Build history of the part. All positions in model axes, mm. A direction names the side the tool comes from. Coordinates: 2 decimals unless noted, no trailing zeros. Order: outer loops, then holes, each group sorted by start corner. A loop starts at its lowest first (then second) coordinate and runs counter-clockwise, first axis right, second up. Notation, with made-up numbers: (80.25, 84) -> (94.25, 84) arc R21 cw to (94.25, 91) -> close; hole circle Ø9 at (82.25, 81). An arc over 180 degrees is marked (long way). Write each question's results on one line, items separated by ' | '.
from build123d import *

# Parameters (mm, degrees)
F0_W         = 6
F0_H         = 10
F1_DEPTH     = 8
F2_T         = 1.2
F3_T1_DEPTH  = 6
F3_T3_DEPTH  = 10
F3_T9_DEPTH  = 8.2404819853
F3_T13_DEPTH = 12.2404819853
F3_T20_DEPTH = 8.2404819853
F3_T24_DEPTH = 12.2404819853
F3_T31_DEPTH = 12.2404819853
F3_T35_DEPTH = 8.2404819853
F3_T42_DEPTH = 8.2404819853
F3_T46_DEPTH = 12.2404819853


# Not quite as in the source:
# - a fillet or chamfer that OpenCascade refuses, or shapes differently, is made with other operations: its cross-section is extruded or revolved along the edge and cut away or added


with BuildPart() as f1:
    # F0 (on Top) → F1 (new body)
    with BuildSketch(Plane.XY):
        Rectangle(F0_W, F0_H)
    extrude(amount=F1_DEPTH)

    # F2
    f2_openings = [f1.faces().sort_by_distance(p)[0] for p in [
        (0, 0, 8),
    ]]
    offset(amount=F2_T, openings=f2_openings, kind=Kind.INTERSECTION)

    # F3: chamfer of 0.5 x 0.8660254038 on 4 edges, made by hand

    # F3_s2 → F3_t1 (cut)
    with BuildSketch(Plane.YZ.offset(-3)):
        Polygon((5, 7.1339745962), (5.5, 8), (5, 8), align=None)
        Polygon((-5, 7.1339745962), (-5.5, 8), (-5, 8), align=None)
    extrude(amount=F3_T1_DEPTH, mode=Mode.SUBTRACT)

    # F3_s4 → F3_t3 (cut)
    with BuildSketch(Plane.XZ.offset(-5)):
        Polygon((-3, 7.1339745962), (-3.5, 8), (-3, 8), align=None)
        Polygon((3, 7.1339745962), (3.5, 8), (3, 8), align=None)
    extrude(amount=F3_T3_DEPTH, mode=Mode.SUBTRACT)


with BuildPart() as f3_tool7:
    # F3_s8 → F3_t9 (new body)
    with BuildSketch(Plane.YZ.offset(5.2404819853)):
        Polygon((5, 7.1339745962), (5.5, 8), (5, 8), align=None)
    extrude(amount=-F3_T9_DEPTH)

    split(bisect_by=Plane.YZ.offset(3), keep=Keep.TOP)


with BuildPart() as f3_tool11:
    # F3_s12 → F3_t13 (new body)
    with BuildSketch(Plane.XZ.offset(5)):
        Polygon((3, 7.1339745962), (3.5, 8), (3, 8), align=None)
    extrude(amount=-F3_T13_DEPTH)

    split(bisect_by=Plane.XZ.offset(-5), keep=Keep.BOTTOM)


with BuildPart() as f3_tool7_1:
    add(f3_tool7.part)

    # F3_t15: intersect F3_tool11
    add(f3_tool11.part, mode=Mode.INTERSECT)


with BuildPart() as f1_1:
    add(f1.part)

    # F3_t5: cut F3_tool7
    add(f3_tool7_1.part, mode=Mode.SUBTRACT)


with BuildPart() as f3_tool18:
    # F3_s19 → F3_t20 (new body)
    with BuildSketch(Plane.YZ.offset(3)):
        Polygon((5, 7.1339745962), (5.5, 8), (5, 8), align=None)
    extrude(amount=-F3_T20_DEPTH)

    split(bisect_by=Plane.YZ.offset(-3), keep=Keep.BOTTOM)


with BuildPart() as f3_tool22:
    # F3_s23 → F3_t24 (new body)
    with BuildSketch(Plane.XZ.offset(-7.2404819853)):
        Polygon((-3, 7.1339745962), (-3.5, 8), (-3, 8), align=None)
    extrude(amount=F3_T24_DEPTH)

    split(bisect_by=Plane.XZ.offset(-5), keep=Keep.BOTTOM)


with BuildPart() as f3_tool18_1:
    add(f3_tool18.part)

    # F3_t26: intersect F3_tool22
    add(f3_tool22.part, mode=Mode.INTERSECT)


with BuildPart() as f1_2:
    add(f1_1.part)

    # F3_t16: cut F3_tool18
    add(f3_tool18_1.part, mode=Mode.SUBTRACT)


with BuildPart() as f3_tool29:
    # F3_s30 → F3_t31 (new body)
    with BuildSketch(Plane.XZ.offset(-5)):
        Polygon((-3, 7.1339745962), (-3.5, 8), (-3, 8), align=None)
    extrude(amount=F3_T31_DEPTH)

    split(bisect_by=Plane.XZ.offset(5), keep=Keep.TOP)


with BuildPart() as f3_tool33:
    # F3_s34 → F3_t35 (new body)
    with BuildSketch(Plane.YZ.offset(-5.2404819853)):
        Polygon((-5, 7.1339745962), (-5.5, 8), (-5, 8), align=None)
    extrude(amount=F3_T35_DEPTH)

    split(bisect_by=Plane.YZ.offset(-3), keep=Keep.BOTTOM)


with BuildPart() as f3_tool29_1:
    add(f3_tool29.part)

    # F3_t37: intersect F3_tool33
    add(f3_tool33.part, mode=Mode.INTERSECT)


with BuildPart() as f1_3:
    add(f1_2.part)

    # F3_t27: cut F3_tool29
    add(f3_tool29_1.part, mode=Mode.SUBTRACT)


with BuildPart() as f3_tool40:
    # F3_s41 → F3_t42 (new body)
    with BuildSketch(Plane.YZ.offset(-3)):
        Polygon((-5, 7.1339745962), (-5.5, 8), (-5, 8), align=None)
    extrude(amount=F3_T42_DEPTH)

    split(bisect_by=Plane.YZ.offset(3), keep=Keep.TOP)


with BuildPart() as f3_tool44:
    # F3_s45 → F3_t46 (new body)
    with BuildSketch(Plane.XZ.offset(7.2404819853)):
        Polygon((3, 7.1339745962), (3.5, 8), (3, 8), align=None)
    extrude(amount=-F3_T46_DEPTH)

    split(bisect_by=Plane.XZ.offset(5), keep=Keep.TOP)


with BuildPart() as f3_tool40_1:
    add(f3_tool40.part)

    # F3_t48: intersect F3_tool44
    add(f3_tool44.part, mode=Mode.INTERSECT)


with BuildPart() as f1_4:
    add(f1_3.part)

    # F3_t38: cut F3_tool40
    add(f3_tool40_1.part, mode=Mode.SUBTRACT)


solid = f1_4.part
Item 1: Pin check, flat tip, straight feed: pin 1 (1.8 mm diameter, centred on x = 1, y = -1.5, fed in from +Z). Stop position of the tip, or through.
Answer:
pin 1: stops at z = 0
Item 2: Slice it at A-A, the plane z = 5.25. List the corners of the cut face in (x, y).
Answer:
outline: (-4.2, -6.2) -> (4.2, -6.2) -> (4.2, 6.2) -> (-4.2, 6.2) -> close; hole (-3, -5) -> (3, -5) -> (3, 5) -> (-3, 5) -> close
Item 3: Drill centre lines: line 1 (X direction, y = 0.25, z = 3); line 2 (Y direction, x = 2, z = 6.5); line 3 (Z direction, x = 2.75, y = 1.5). Where is each one in solid material? Low to high. Write a range as from..to.
Answer:
line 1: x = -4.2..-3, 3..4.2 | line 2: y = -6.2..-5, 5..6.2 | line 3: z = -1.2..0
Item 4: Slice it at B-B, the plane x = -2.25. List the corners of the cut face in (y, z).
Answer:
outline: (-6.2, -1.2) -> (6.2, -1.2) -> (6.2, 8) -> (5.5, 8) -> (5, 7.13) -> (5, 0) -> (-5, 0) -> (-5, 7.13) -> (-5.5, 8) -> (-6.2, 8) -> close
Item 5: Slice it at C-C, the plane y = -4. List the corners of the cut face in (x, z), and give its area (3 significant figures).
Answer:
outline: (-4.2, -1.2) -> (4.2, -1.2) -> (4.2, 8) -> (3.5, 8) -> (3, 7.13) -> (3, 0) -> (-3, 0) -> (-3, 7.13) -> (-3.5, 8) -> (-4.2, 8) -> close | area: 28.8 mm^2
Item 6: Tool access for faces 1 (the flat face through (4.2, 0, 3)), 2 (the flat face through (0, 0, 0)): list every direction of +Z, -Z, +X, -X, +Y, -Y with a clear straight run to the whole face (end or side of a thin tool).
Answer:
face 1: +Z, -Z, +X, +Y, -Y | face 2: +Z
Item 7: Pull direction Y, two halves, no side cores. Call faces 3 (the flat face through (0, -6.2, 3)), 4 (the flat face through (-4.2, 0, 3)), 5 (the flat face through (-0.049, 5.246, 7.561)), 6 (the flat face through (0, 6.2, 3)): released by +Y, released by -Y, zero draft, split by the parting line, or undercut.
Answer:
face 3: released by -Y | face 4: zero draft | face 5: undercut | face 6: released by +Y
